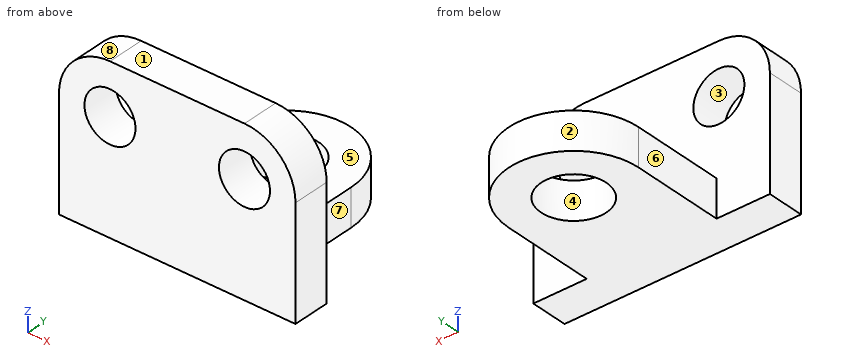
from build123d import *

# Parameters (mm, degrees)
SKETCH_1_R      = 5.5
EXTRUDE_1_DEPTH = 8
SKETCH_2_R      = 7
EXTRUDE_2_DEPTH = 8


with BuildPart() as part:
    # 草图1 → 凸台-拉伸1 (new body)
    with BuildSketch(Plane(origin=(0, 0, 0), x_dir=(1, 0, 0), z_dir=(0, 1, 0))):
        with BuildLine():
            Line((-14.5, -17.5), (14.5, -17.5))
            ThreePointArc((14.5, -17.5), (22.278174593, -14.278174593), (25.5, -6.5))
            Line((25.5, -6.5), (25.5, 17.5))
            Line((25.5, 17.5), (-25.5, 17.5))
            Line((-25.5, 17.5), (-25.5, -6.5))
            ThreePointArc((-25.5, -6.5), (-22.278174593, -14.278174593), (-14.5, -17.5))
        make_face()
        with Locations(Location((14.5, -6.5, 0), (0, 0, 270))):
            Circle(SKETCH_1_R, mode=Mode.SUBTRACT)
        with Locations(Location((-14.5, -6.5, 0), (0, 0, 90))):
            Circle(SKETCH_1_R, mode=Mode.SUBTRACT)
    extrude(amount=EXTRUDE_1_DEPTH)

    # 草图2 → 凸台-拉伸2 (add)
    with BuildSketch(Plane(origin=(0, 0, -17.5), x_dir=(-1, 0, 0), z_dir=(0, 0, -1))):
        with BuildLine():
            Line((-14, 8), (14, 8))
            Line((14, 8), (14, 28))
            ThreePointArc((14, 28), (0, 42), (-14, 28))
            Line((-14, 28), (-14, 8))
        make_face()
        with Locations((0, 28)):
            Circle(SKETCH_2_R, mode=Mode.SUBTRACT)
    extrude(amount=-EXTRUDE_2_DEPTH)


solid = part.part
Could you check a few things on this model? Use its own coordinates, in mm. Face numbers are marked on the shaded views. A direction names the side the tool comes from. Round coordinates to 2 decimals unless told otherwise and drop trailing zeros. Write each loop counter-clockwise with the first axis right and the second up, starting at its lowest first coordinate (ties: lowest second). Pieces come first, ordered by that corner, then holes. Notation, with made-up numbers: (37, 40) - (48, 40) arc R24 cw to (48, 56) - close; hole circle Ø10 at (-35, 20). An arc over 180 degrees is marked (long way). Use a Markdown table: item, result.
Q1. I want a section at A-A (x = 0). List the corners of the cut face in (y, z) for me.
Output values:
| item | result |
|---|---|
| outline | (0, -17.5) - (21, -17.5) - (21, -9.5) - (8, -9.5) - (8, 17.5) - (0, 17.5) - close; (35, -17.5) - (42, -17.5) - (42, -9.5) - (35, -9.5) - close |
Q2. For pin 1 (17.5 mm diameter, centred on x = -9, z = 7, fed in from +Y); pin 2 (22.5 mm diameter, centred on x = 4.5, y = 31.5, fed in from +Z); pin 3 (9 mm diameter, centred on y = 21, z = -14, fed in from +X), each with a flat end and sliding along its axis, tell me the tip position at first contact or that it passes through.
Output values:
| item | result |
|---|---|
| pin 1 | y = 8 |
| pin 2 | z = -9.5 |
| pin 3 | x = 14 |
Q3. I want a section at B-B (y = 5). List the corners of the cut face in (x, z) for me.
Output values:
| item | result |
|---|---|
| outline | (-25.5, -17.5) - (25.5, -17.5) - (25.5, 6.5) arc R11 ccw to (14.5, 17.5) - (-14.5, 17.5) arc R11 ccw to (-25.5, 6.5) - close; hole circle Ø11 at (-14.5, 6.5); hole circle Ø11 at (14.5, 6.5) |
Q4. Thinking about a two-plate mould opening in X: for the marked faces 1, 2, 3 and 4, which applies, released by +X, released by -X, zero draft, split by the parting line, or undercut?
Output values:
| item | result |
|---|---|
| face 1 | zero draft |
| face 2 | split by the parting line |
| face 3 | undercut |
| face 4 | undercut |
Q5. I want a section at D-D (y = 33). List the corners of the cut face in (x, z) for me.
Output values:
| item | result |
|---|---|
| outline | (-13.08, -17.5) - (-4.9, -17.5) - (-4.9, -9.5) - (-13.08, -9.5) - close; (4.9, -17.5) - (13.08, -17.5) - (13.08, -9.5) - (4.9, -9.5) - close |
Q6. I want a section at C-C (z = 5). List the corners of the cut face in (x, y) for me.
Output values:
| item | result |
|---|---|
| outline | (-25.5, 0) - (-19.79, 0) - (-19.79, 8) - (-25.5, 8) - close; (-9.21, 0) - (9.21, 0) - (9.21, 8) - (-9.21, 8) - close; (19.79, 0) - (25.5, 0) - (25.5, 8) - (19.79, 8) - close |
Q7. Please list where these lines run through material, in increasing order: L1, parallel to X at y = 6, z = 6.5; L2, parallel to X at y = 5.5, z = 10; L3, parallel to Y at x = 0, z = -11.25.
Output values:
| item | result |
|---|---|
| L1 | -25.5 to -20, -9 to 9, 20 to 25.5 |
| L2 | -24.93 to -18.74, -10.26 to 10.26, 18.74 to 24.93 |
| L3 | 0 to 21, 35 to 42 |
Q8. For the marked faces 5, 6, 7 and 8, which set-ups out of +Z, -Z, +X, -X, +Y, -Y let a thin tool reach every point of the face, with its end or its side?
Output values:
| item | result |
|---|---|
| face 5 | +Z, +X, -X, +Y |
| face 6 | +Z, -Z, -X, +Y |
| face 7 | +Z, -Z, +X, +Y |
| face 8 | +Z, -X, +Y, -Y |
